from build123d import *

# Parameters (mm, degrees)
SKETCH_1_R          = 1.5
EXTRUDE_1_DEPTH     = 4
EXTRUDE_2_DEPTH     = 20.84
EXTRUDE_START       = -4
EXTRUDE_3_DEPTH     = 4
CUT_EXTRUDE_START   = -20.84
CUT_EXTRUDE_1_DEPTH = 20.84
SKETCH_15_R         = 1.5
CUT_EXTRUDE_2_DEPTH = 86.104469456


# Read off the part's stored shape, not the designer's step: the extrude step
with BuildPart() as part:
    # Sketch 1 → Extrude 1 (new body)
    with BuildSketch(Plane.XY):
        with BuildLine():
            Line((-8.883361298, 38.430372232), (-10.42356995, 28.043950456))
            ThreePointArc((-10.42356995, 28.043950456), (-10.775128008, 27.17392517), (-11.484802252, 26.560003729))
            ThreePointArc((-11.484802252, 26.560003729), (-13.893149851, 24.653752275), (-15.405733358, 21.980547476))
            ThreePointArc((-15.405733358, 21.980547476), (-20.465380085, 19.450724806), (-22.995202754, 24.510371532))
            Line((-22.995202754, 24.510371532), (-18.451197233, 38.142383115))
            ThreePointArc((-18.451197233, 38.142383115), (-18.348830032, 38.742204214), (-18.431570381, 39.345046174))
            Line((-18.431570381, 39.345046174), (-22.233001172, 52.125165651))
            ThreePointArc((-22.233001172, 52.125165651), (-22.31526172, 52.64074939), (-22.261276417, 53.160055635))
            Line((-22.261276417, 53.160055635), (-18.372774426, 69.438220218))
            ThreePointArc((-18.372774426, 69.438220218), (-18.096529541, 70.075517478), (-17.618975762, 70.579899696))
            Line((-17.618975762, 70.579899696), (-6.150614111, 79.086205979))
            ThreePointArc((-6.150614111, 79.086205979), (-5.627950875, 79.131232586), (-5.352746621, 78.684615443))
            Line((-5.352746621, 78.684615443), (-5.352746621, 75.677999772))
            ThreePointArc((-5.352746621, 75.677999772), (-14.888864346, 58.677248629), (-9.31952103, 39.997165768))
            ThreePointArc((-9.31952103, 39.997165768), (-8.934989705, 39.260105305), (-8.883361298, 38.430372232))
        make_face()
        with Locations(Location((-19.200468056, 23.245459504, 0), (0, 0, 180))):
            Circle(SKETCH_1_R, mode=Mode.SUBTRACT)
        with Locations((-14.200468056, 38.245459504)):
            Circle(SKETCH_1_R, mode=Mode.SUBTRACT)
    extrude(amount=EXTRUDE_1_DEPTH)

    # Sketch 9 → Extrude 2 (add)
    with BuildSketch(Plane(origin=(0, 0, 0), x_dir=(-1, 0, 0), z_dir=(0, 0, -1))):
        with BuildLine():
            Line((18.431570381, 39.345046174), (11.995527079, 43.954984078))
            ThreePointArc((11.995527079, 43.954984078), (14.51123125, 61.038775991), (5.352746621, 75.677999772))
            Line((5.352746621, 75.677999772), (5.352746621, 78.684615443))
            ThreePointArc((5.352746621, 78.684615443), (5.627950875, 79.131232586), (6.150614111, 79.086205979))
            Line((6.150614111, 79.086205979), (17.618975762, 70.579899696))
            ThreePointArc((17.618975762, 70.579899696), (18.096529541, 70.075517478), (18.372774426, 69.438220218))
            Line((18.372774426, 69.438220218), (22.261276417, 53.160055635))
            ThreePointArc((22.261276417, 53.160055635), (22.31526172, 52.64074939), (22.233001172, 52.125165651))
            Line((22.233001172, 52.125165651), (18.431570381, 39.345046174))
        make_face()
    extrude(amount=-EXTRUDE_2_DEPTH)

    # Sketch 13 → Extrude 3 (add)
    with BuildSketch(Plane.XY.offset(20.84).offset(EXTRUDE_START)):
        with BuildLine():
            Line((-11.995527079, 43.954984078), (-18.431570381, 39.345046174))
            ThreePointArc((-18.431570381, 39.345046174), (-18.348830032, 38.742204214), (-18.451197233, 38.142383115))
            Line((-18.451197233, 38.142383115), (-22.995202754, 24.510371532))
            ThreePointArc((-22.995202754, 24.510371532), (-20.465380085, 19.450724806), (-15.405733358, 21.980547476))
            ThreePointArc((-15.405733358, 21.980547476), (-13.893149851, 24.653752275), (-11.484802252, 26.560003729))
            ThreePointArc((-11.484802252, 26.560003729), (-10.775128008, 27.17392517), (-10.42356995, 28.043950456))
            Line((-10.42356995, 28.043950456), (-8.883361298, 38.430372232))
            ThreePointArc((-8.883361298, 38.430372232), (-8.934989705, 39.260105305), (-9.31952103, 39.997165768))
            ThreePointArc((-9.31952103, 39.997165768), (-10.752284945, 41.91200409), (-11.995527079, 43.954984078))
        make_face()
    extrude(amount=EXTRUDE_3_DEPTH)

    # Cut-Extrude 1 outline → Cut-Extrude 1 (cut)
    with BuildSketch(Plane(origin=(0, 0, 0), x_dir=(-1, 0, 0), z_dir=(0, 0, -1)).offset(CUT_EXTRUDE_START)):
        with BuildLine():
            ThreePointArc((12.745402307, 38.62665484), (15.654449874, 37.860150418), (12.747581778, 38.634879176))
            ThreePointArc((12.747581778, 38.634879176), (12.750516716, 38.629700459), (12.745402307, 38.62665484))
        make_face()
    extrude(amount=CUT_EXTRUDE_1_DEPTH, mode=Mode.SUBTRACT)

    # Sketch 15 → Cut-Extrude 2 (cut, through all)
    with BuildSketch(Plane(origin=(0, 0, 0), x_dir=(-1, 0, 0), z_dir=(0, 0, -1))):
        with Locations((19.200468056, 23.245459504)):
            Circle(SKETCH_15_R)
    extrude(amount=-CUT_EXTRUDE_2_DEPTH, mode=Mode.SUBTRACT)


solid = part.part
Geometry: final body of the model. Coordinates: model frame, mm. A direction names the side the tool comes from. Round coordinates to 2 decimals unless told otherwise and drop trailing zeros. Loops run counter-clockwise (first coordinate to the right, second up) from the corner with the lowest first, then second, coordinate; pieces in that order, holes last. Notation, with made-up numbers: (41, 51.25) - (63, 51.25) arc R22 ccw to (63, 67.25) - close; hole circle Ø1 at (84.25, 6.5). An arc over 180 degrees is marked (long way). Write each question's results on one line, items separated by ' | '. Start each with the question number.
1) Cut plane C-C on x = -19.75. Return loops of the section in (y, z), then the cut area to 3 significant figures.
2) Access query for faces 4 (the face through (-20.7, 31.4, 18.8)), 5 (the face through (-10.783, 27.163, 18.812)). Directions: +Z, -Z, +X, -X, +Y, -Y. A direction counts if a zero-diameter tool reaches every point of the face in a straight line with its end or side. Return the directions, or none.
3) Mould query, pull axis X, two halves, no side actions, for faces 1 (the face through (-20.586, 23.82, 1.972)), 2 (the face through (-13.86, 24.69, 1.97)), 3 (the face through (-20.306, 45.646, 10.274)). Classes: released by +X, released by -X, zero draft, split by the parting line, or undercut.
4) Cut plane B-B on z = 19.25. Count the separate pieces of the cut face and the enclosed holes in it, then the cut area to 3 significant figures.
5) Line query: probe 1 along Z at (x, y) = (-10.5, 37); probe 2 along Y at (x, z) = (-7.75, 10.75); probe 3 along Y at (x, z) = (-11, 3.75). Output: solid intervals per line, ascending. Write a range as [from, to].
6) Cut plane A-A on y = 34.5. Return loops of the section in (x, z).
7) Cut plane D-D on z = 13.25. Return loops of the section in (x, y), then the cut area to 3 significant figures.
8) First-contact query: P1, Ø3, axis at x = -8.5, z = 12.5, coming from the -Y side; P2, Ø10, axis at y = 28.5, z = 15.5, coming from the +X side; P3, Ø3, axis at x = -18, z = 14, coming from the -Y side. Flat tips, straight axial feed; report the tip coordinate or a pass-through.
Verdict:
1) outline: (19.28, 0) - (21.85, 0) - (21.85, 4) - (19.28, 4) - close; (19.28, 16.84) - (21.85, 16.84) - (21.85, 20.84) - (19.28, 20.84) - close; (24.64, 0) - (34.25, 0) - (34.25, 4) - (24.64, 4) - close; (24.64, 16.84) - (34.25, 16.84) - (34.25, 20.84) - (24.64, 20.84) - close; (43.78, 0) - (63.67, 0) - (63.67, 20.84) - (43.78, 20.84) - close | area: 512 mm2
2) face 4: +Z, -Z, -X | face 5: +Z, -Z, +X, -Y
3) face 1: undercut | face 2: released by +X | face 3: released by -X
4) separate pieces: 1 | enclosed holes: 2 | area: 437 mm2
5) probe 1: z = [0, 4], [16.84, 20.84] | probe 2: y = [73.56, 77.9] | probe 3: y = [26.91, 42.29], [69.54, 75.49]
6) outline: (-19.67, 0) - (-9.47, 0) - (-9.47, 4) - (-19.67, 4) - close; (-19.67, 16.84) - (-9.47, 16.84) - (-9.47, 20.84) - (-19.67, 20.84) - close
7) outline: (-22.26, 53.16) arc R2 ccw to (-22.23, 52.13) - (-18.43, 39.35) - (-12, 43.95) arc R25 cw to (-5.35, 75.68) - (-5.35, 78.68) arc R0.5 ccw to (-6.15, 79.09) - (-17.62, 70.58) arc R2 ccw to (-18.37, 69.44) - close | area: 240 mm2
8) P1: stops at y = 70.97 | P2: stops at x = -9.64 | P3: stops at y = 39.35
